```python
from build123d import *

# Parameters (mm, degrees)
F0_R     = 12.5
F1_DEPTH = 510
F2_W     = 71.5121626854
F2_H     = 186.2277984619
F2_W_2   = 42.5452291965
F2_H_2   = 161.7869436741
F2_W_3   = 31.6825956106
F2_H_3   = 140.0617212057
F2_W_4   = 24.440869689
F2_H_4   = 119.2417219281
F2_W_5   = 87.8060813993
F2_H_5   = 154.5452028513
F2_W_6   = 63.3652210236
F2_H_6   = 150.9243249893
F2_W_7   = 11.7678269744
F2_H_7   = 87.5591114163
F2_W_8   = 19.9147760868
F2_H_8   = 90.2747660875
F2_W_9   = 18.1043446064
F2_H_9   = 86.6538956761


with BuildPart() as f1:
    # F0 (on Right) → F1 (new body, symmetric)
    with BuildSketch(Plane.YZ):
        Circle(F0_R)
    extrude(amount=F1_DEPTH, both=True)

    # F2 (on Top) → F3 (revolve)
    with BuildSketch(Plane.XY):
        with Locations((391.5624916553, 93.113899231)):
            Rectangle(F2_W, F2_H)
        with Locations((-370.6304728985, 93.113899231)):
            Rectangle(F2_W, F2_H)
        with Locations((-272.8670090437, 80.893471837)):
            Rectangle(F2_W_2, F2_H_2)
        with Locations((-207.6913639903, 70.0308606029)):
            Rectangle(F2_W_3, F2_H_3)
        with Locations((-144.3261578679, 59.6208609641)):
            Rectangle(F2_W_4, F2_H_4)
        with Locations((-22.121806629, 77.2726014256)):
            Rectangle(F2_W_5, F2_H_5)
        with Locations((119.5446997881, 75.4621624947)):
            Rectangle(F2_W_6, F2_H_6)
        with Locations((223.1920994818, 43.7795557082)):
            Rectangle(F2_W_7, F2_H_7)
        with Locations((264.3794864416, 45.1373830438)):
            Rectangle(F2_W_8, F2_H_8)
        with Locations((306.0194700956, 43.3269478381)):
            Rectangle(F2_W_9, F2_H_9)
    revolve(axis=Axis((10.4660093784, 0, 0), (1, 0, 0)))


solid = f1.part
```
Source: CAD feature listing. Evaluate the final solid. Frame: model axes, mm. A direction names the side the tool comes from. Round coordinates to 2 decimals unless told otherwise and drop trailing zeros. Order: outer loops, then holes, each group sorted by start corner. A loop starts at its lowest first (then second) coordinate and runs counter-clockwise, first axis right, second up. Notation, with made-up numbers: (31.5, 87) -> (48.5, 87) arc R17 ccw to (48.5, 108) -> close; hole circle Ø9 at (29, 47.25). An arc over 180 degrees is marked (long way). Use CSV: the item, a comma, the result in double quotes.
(1) Section A-A on z = 103. Return the cut outline in (x, y).
Report:
outline,"(-406.39, -155.15) -> (-334.87, -155.15) -> (-334.87, 155.15) -> (-406.39, 155.15) -> close; (-294.14, -124.76) -> (-251.59, -124.76) -> (-251.59, 124.76) -> (-294.14, 124.76) -> close; (-223.53, -94.91) -> (-191.85, -94.91) -> (-191.85, 94.91) -> (-223.53, 94.91) -> close; (-156.55, -60.08) -> (-132.11, -60.08) -> (-132.11, 60.08) -> (-156.55, 60.08) -> close; (-66.02, -115.22) -> (21.78, -115.22) -> (21.78, 115.22) -> (-66.02, 115.22) -> close; (87.86, -110.31) -> (151.23, -110.31) -> (151.23, 110.31) -> (87.86, 110.31) -> close; (355.81, -155.15) -> (427.32, -155.15) -> (427.32, 155.15) -> (355.81, 155.15) -> close"
(2) Section B-B on x = 443. Return the cut outline in (y, z), and give its area (3 significant figures).
Report:
outline,"circle Ø25 at (0, 0)"
area,"491 mm^2"
(3) Ray query, L1, parallel to X at y = 103, z = 63.5; L2, parallel to X at y = -147, z = -12; L3, parallel to X at y = -115.5, z = -127.5. Return the intervals inside material, ascending.
Report:
L1,"-406.39 to -334.87, -294.14 to -251.59, -223.53 to -191.85, -66.02 to 21.78, 87.86 to 151.23, 355.81 to 427.32"
L2,"-406.39 to -334.87, -294.14 to -251.59, -66.02 to 21.78, 87.86 to 151.23, 355.81 to 427.32"
L3,"-406.39 to -334.87, 355.81 to 427.32"
(4) Access query for faces 4 (the face through (469.238, 11.923, 3.755)), 5 (the face through (285.81, 11.923, 3.755)). Directions: +Z, -Z, +X, -X, +Y, -Y. A direction counts if a zero-diameter tool reaches every point of the face in a straight line with its end or side. Return the directions, or none.
Report:
face 4,"+X"
face 5,"none"
(5) First-contact query: pin 1 Ø6 at (y, z) = (-97.5, -25) entering from +X; pin 2 Ø2 at (x, z) = (87, -20) entering from +Y; pin 3 Ø1.5 at (x, z) = (91.5, 95.5) entering from -Y. Flat tips, straight axial feed; report the tip coordinate or a pass-through.
Report:
pin 1,"x = 427.32"
pin 2,"y = 149.66"
pin 3,"y = -117.48"
(6) Section C-C on z = 26. Count the separate pieces of the cut face and the enclosed holes in it, and give its area (3 significant figures).
Report:
separate pieces,"10"
enclosed holes,"0"
area,"135,000 mm^2"
(7) Pull-direction query (X, two-part tool) for faces 1 (the face through (229.076, 1, -18)), 2 (the face through (-207.47, 64.63, -124.26)), 3 (the face through (-457.468, 11.923, 3.755)); classes: +X half, -X half, draft (parallel to the pull), parting line (faces both ways), or undercut.
Report:
face 1,"undercut"
face 2,"undercut"
face 3,"draft"
